Geometry check sheet. Reference: the model listing, model coordinates, mm. Face numbers are marked on the shaded views. A direction names the side the tool comes from. Give positions to 0.01 mm unless a question says otherwise; leave off trailing zeros. Write each loop counter-clockwise with the first axis right and the second up, starting at its lowest first coordinate (ties: lowest second). Pieces come first, ordered by that corner, then holes. Notation, with made-up numbers: (-26.75, 13.25) -> (-20.75, 13.25) arc R11 ccw to (-20.75, 34.25) -> close; hole circle Ø1 at (39, 53). An arc over 180 degrees is marked (long way). Use a Markdown table: item, result. Add a question column.
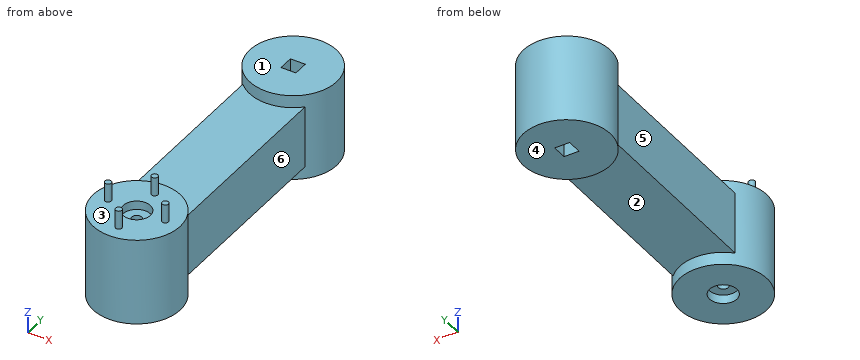
from build123d import *

# Parameters (mm, degrees)
CROQUIS1_R              = 35
SALIENTE_EXTRUIR1_DEPTH = 70
CROQUIS2_W              = 50
CROQUIS2_H              = 50
SALIENTE_EXTRUIR2_DEPTH = 200
CROQUIS4_R              = 35
SALIENTE_EXTRUIR4_DEPTH = 70
CROQUIS5_R              = 4
CORTAR_EXTRUIR1_DEPTH   = 150
CROQUIS6_R              = 11
CORTAR_EXTRUIR3_DEPTH   = 7
CORTAR_EXTRUIR4_START   = -7
CROQUIS7_R              = 11
CORTAR_EXTRUIR4_DEPTH   = 7
CROQUIS8_R              = 2.5
SALIENTE_EXTRUIR5_DEPTH = 15
CROQUIS9_W              = 12
CROQUIS9_H              = 12
CORTAR_EXTRUIR5_DEPTH   = 152


with BuildPart() as part:
    # Croquis1 → Saliente-Extruir1 (new body)
    with BuildSketch(Plane.XY):
        Circle(CROQUIS1_R)
    extrude(amount=SALIENTE_EXTRUIR1_DEPTH)

    # Croquis2 → Saliente-Extruir2 (add)
    with BuildSketch(Plane(origin=(0, 0, 0), x_dir=(1, 0, 0), z_dir=(0, 1, 0))):
        with Locations((0, -35)):
            Rectangle(CROQUIS2_W, CROQUIS2_H)
    extrude(amount=SALIENTE_EXTRUIR2_DEPTH)

    # Croquis4 → Saliente-Extruir4 (add)
    with BuildSketch(Plane.XY):
        with Locations((0, 200)):
            Circle(CROQUIS4_R)
    extrude(amount=SALIENTE_EXTRUIR4_DEPTH)

    # Croquis5 → Cortar-Extruir1 (cut)
    with BuildSketch(Plane.XY):
        Circle(CROQUIS5_R)
    extrude(amount=CORTAR_EXTRUIR1_DEPTH, mode=Mode.SUBTRACT)

    # Croquis6 → Cortar-Extruir3 (cut)
    with BuildSketch(Plane.XY):
        Circle(CROQUIS6_R)
    extrude(amount=CORTAR_EXTRUIR3_DEPTH, mode=Mode.SUBTRACT)

    # Croquis7 → Cortar-Extruir4 (cut)
    with BuildSketch(Plane.XY.offset(70).offset(CORTAR_EXTRUIR4_START)):
        Circle(CROQUIS7_R)
    extrude(amount=CORTAR_EXTRUIR4_DEPTH, mode=Mode.SUBTRACT)

    # Croquis8 → Saliente-Extruir5 (add)
    with BuildSketch(Plane.XY.offset(70)):
        with Locations((-23, 0)):
            Circle(CROQUIS8_R)
        with Locations((0, -23)):
            Circle(CROQUIS8_R)
        with Locations((23, 0)):
            Circle(CROQUIS8_R)
        with Locations((0, 23)):
            Circle(CROQUIS8_R)
    extrude(amount=SALIENTE_EXTRUIR5_DEPTH)

    # Croquis9 → Cortar-Extruir5 (cut)
    with BuildSketch(Plane.XY.offset(70)):
        with Locations((0, 200)):
            Rectangle(CROQUIS9_W, CROQUIS9_H)
    extrude(amount=-CORTAR_EXTRUIR5_DEPTH, mode=Mode.SUBTRACT)


solid = part.part
1) Sectioned sample at B-B, the plane z = 44.5. Enter the section's corners in (x, y).
2) Tool access check on the marked faces 3, 4, 5 and 6. Record the directions out of +Z, -Z, +X, -X, +Y, -Y that give a thin tool (end or side, any length) a straight path to the whole face; none if there is none.
3) Gauge pin test, flat ends, axial feed: P1, Ø25, axis at x = -4.5, y = 78.5, coming from the +Z side; P2, Ø17.5, axis at x = 0, y = 0, coming from the -Z side; P3, Ø2, axis at x = -13.5, z = 23.5, coming from the +Y side. Record the tip position at first contact, or that the pin passes through.
4) Sectioned sample at C-C, the plane x = -29.5. Enter the section's corners in (y, z).
5) Sectioned sample at D-D, the plane z = 77. Enter the section's corners in (x, y).
6) Material ranges on probe 1 along Y at (x, z) = (0, 67); probe 2 along X at (y, z) = (198, 38); probe 3 along Z at (x, y) = (6.5, 126), recorded low to high. Write a range as [from, to].
7) Draft check along Y on the marked faces 1 and 2. Enter one of: +Y half, -Y half, draft (parallel to the pull), parting line (faces both ways), or undercut.
8) Sectioned sample at A-A, the plane y = 0. Enter the section's corners in (x, z).
Check values:
| question | item | result |
|---|---|---|
| 1 | outline | (-25, 24.49) arc R35 ccw (long way) to (25, 24.49) -> (25, 175.51) arc R35 ccw (long way) to (-25, 175.51) -> close; hole (-6, 194) -> (6, 194) -> (6, 206) -> (-6, 206) -> close; hole circle Ø8 at (0, 0) |
| 2 | face 3 | +Z |
| 2 | face 4 | -Z, +X, -X, +Y, -Y |
| 2 | face 5 | +Z, -Z, -X |
| 2 | face 6 | +Z, -Z, +X |
| 3 | P1 | z = 60 |
| 3 | P2 | z = 7 |
| 3 | P3 | y = 232.69 |
| 4 | outline | (-18.83, 0) -> (18.83, 0) -> (18.83, 70) -> (-18.83, 70) -> close; (181.17, 0) -> (218.83, 0) -> (218.83, 70) -> (181.17, 70) -> close |
| 5 | outline | circle Ø5 at (-23, 0); circle Ø5 at (0, -23); circle Ø5 at (0, 23); circle Ø5 at (23, 0) |
| 6 | probe 1 | [-35, -11], [11, 35], [165, 194], [206, 235] |
| 6 | probe 2 | [-34.94, -6], [6, 34.94] |
| 6 | probe 3 | [10, 60] |
| 7 | face 1 | draft |
| 7 | face 2 | undercut |
| 8 | outline | (-35, 0) -> (-11, 0) -> (-11, 7) -> (-4, 7) -> (-4, 63) -> (-11, 63) -> (-11, 70) -> (-20.5, 70) -> (-20.5, 85) -> (-25.5, 85) -> (-25.5, 70) -> (-35, 70) -> close; (4, 7) -> (11, 7) -> (11, 0) -> (35, 0) -> (35, 70) -> (25.5, 70) -> (25.5, 85) -> (20.5, 85) -> (20.5, 70) -> (11, 70) -> (11, 63) -> (4, 63) -> close |
